Input: part model. Units: mm. Frame: model coordinates. Face numbers are marked on the shaded views. A direction names the side the tool comes from. Give positions to 0.01 mm unless a question says otherwise; leave off trailing zeros. Write each loop counter-clockwise with the first axis right and the second up, starting at its lowest first coordinate (ties: lowest second). Pieces come first, ordered by that corner, then holes.
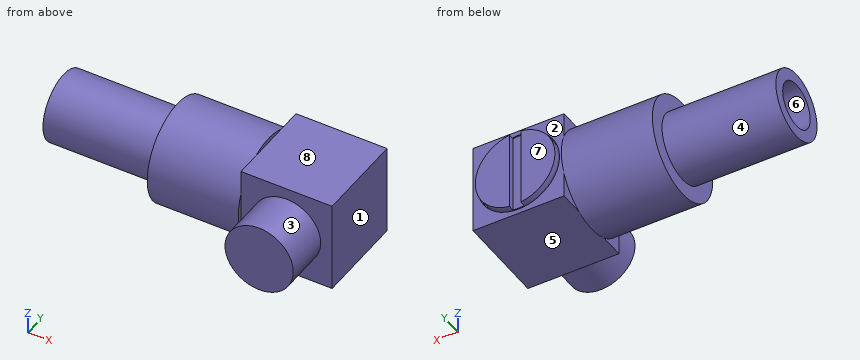
Autodesk Inventor part; units mm, degrees
ref_plane "YZ Plane" through (0, 0, 0) normal (1, 0, 0) x (0, 1, 0)
ref_plane "XZ Plane" through (0, 0, 0) normal (0, 1, 0) x (-1, 0, 0)
ref_plane "XY Plane" through (0, 0, 0) normal (0, 0, 1) x (1, 0, 0)
sketch "Sketch1" plane through (0, 0, 0) normal (0, 1, 0) x (-1, 0, 0)
  line L0 (0, 0) -> (8, 0)
  line L1 (8, 0) -> (8, -4.4)
  line L2 (8, -4.4) -> (0, -4.4)
  line L3 (0, -4.4) -> (0, 0)
  line L4 (0, 0) -> (-8, 0)
  line L5 (-8, 0) -> (-8, -4)
  line L6 (-8, -4) -> (0, -4)
  line L7 (0, -4) -> (0, 0)
  line L8 (-8, 0) -> (0, 0)
  line L9 (0, 0) -> (0, 4)
  line L10 (0, 4) -> (-8, 4)
  line L11 (-8, 4) -> (-8, 0)
  circle A0 centre (-4, 0) radius 3
  line L12 (8, -2) -> (18, -2)
  line L13 (18, -2) -> (18, -3)
  line L14 (18, -3) -> (8, -3)
  line L15 (8, -3) -> (8, -2)
  circle A1 centre (-4, 0) radius 3.5
  line L16 (-3.5, 3.6063) -> (-4.5, 3.6063)
  line L17 (-4.5, 3.6063) -> (-4.5, -3.6063)
  line L18 (-4.5, -3.6063) -> (-3.5, -3.6063)
  line L19 (-3.5, -3.6063) -> (-3.5, 3.6063)
  line L20 (-3.5, 3.6063) -> (-4.5, -3.6063) construction
  line L21 (-4.5, 3.6063) -> (-3.5, -3.6063) construction
  point P0 (-4.5, 3.4641)
  point P1 (-4.5, -3.4641)
  point P2 (-3.5, -3.4641)
  point P3 (-3.5, 3.4641)
  dimension "d0" = 8
  dimension "d1" = 4.4
  dimension "d2" = 8
  dimension "d3" = 4
  dimension "d4" = 4
  dimension "d5" = 6
  dimension "d6" = 10
  dimension "d7" = 1
  dimension "d8" = 2
  dimension "d9" = 7
  dimension "d10" = 1
revolve "Revolution1" add sketch "Sketch1" angle 360 about axis through (0, 0, 0) along (-1, 0, 0) contours L0 L1 L2 L3
revolve "Revolution2" add sketch "Sketch1" angle 360 about axis through (0, 0, 0) along (-1, 0, 0) contours L12 L13 L14 L1
extrude "Extrusion1" add sketch "Sketch1" along normal mid plane 8 contours L3 L6 L5 L4 A1 L17 L18 L19 | L4 A1 L19 L16 L17 L11 L10 L9 | A1 L19 A0 L4 | L4 A0 L19 A1 | A0 L19 L4 | L4 L19 A0 | L19 A0 L17 A1 | A1 L17 L16 L19 | L19 L18 L17 A1 | A1 L17 A0 L19 | L19 A0 L17 L4 | L4 L17 A0 L19 | L17 A0 L4 A1 | A1 L4 A0 L17 | L17 A0 L4 | L4 A0 L17
extrude "Extrusion2" add sketch "Sketch1" against normal blind 8 contours A0 L19 L4 | L4 L19 A0 | L19 A0 L17 L4 | L4 L17 A0 L19 | L17 A0 L4 | L4 A0 L17
extrude "Extrusion3" add sketch "Sketch1" along normal blind 4.5 contours A1 L19 A0 L4 | L4 A0 L19 A1 | A0 L19 L4 | L4 L19 A0 | L17 A0 L4 A1 | A1 L4 A0 L17 | L17 A0 L4 | L4 A0 L17
sketch "Sketch2" plane through (0, 4, 0) normal (0, 1, 0) x (1, 0, 0)
  arc A0 (3.5, 3.4641) -> (3.5, -3.4641) centre (4, 0) ccw
  line L0 (3.5, -3.4641) -> (3.5, 3.4641)
  arc A1 (4.5, -3.4641) -> (4.5, 3.4641) centre (4, 0) ccw
  line L1 (4.5, 3.4641) -> (4.5, -3.4641)
  line L2 (4.5, -3.4641) -> (4.5, 3.4641)
  arc A2 (4.5, -3.4641) -> (4.5, 3.4641) centre (4, 0) ccw
  line L3 (3.5, 3.4641) -> (3.5, -3.4641)
  arc A3 (3.5, 3.4641) -> (3.5, -3.4641) centre (4, 0) ccw
  line L4 (0, -4) -> (8, -4)
  line L5 (8, -4) -> (8, 4)
  line L6 (8, 4) -> (0, 4)
  line L7 (0, 4) -> (0, 1.833)
  line L8 (0, -1.833) -> (0, 1.833)
  line L9 (0, -1.833) -> (0, -4)
  circle A4 centre (4, 0) radius 3.6
  circle A5 centre (4, 0) radius 3.5
  point P0 (0, 0)
  point P1 (3.5, -3.4641)
  dimension "d19" = 7.2
extrude "Extrusion4" cut sketch "Sketch2" against normal blind 0.5 contours A4
thread "Thread1"
properties part number "6mm hose fitting"
Item 1: Ray query, line 1 (Z direction, x = -15.5, y = 0); line 2 (X direction, y = 0, z = 4.25). Return the intervals inside material, ascending.
Item 2: Section A-A (x = 4). Return loops of the section in (y, z), and give its area (3 significant figures).
Item 3: Set-up query: the marked faces 1, 2, 3, 4 and 5. Return all of +Z, -Z, +X, -X, +Y, -Y with unobstructed straight access to the full face (end or side cutting, diameter ignored); none if empty.
Item 4: Section D-D (x = -9.25). Return loops of the section in (y, z).
Item 5: Section C-C (y = 0). Return loops of the section in (x, z).
Item 6: Pin query (flat end, axial travel): pin 1 (1 mm diameter, centred on x = -11, y = 2, fed in from -Z); pin 2 (0.7 mm diameter, centred on y = 3, z = 2.5, fed in from -X); pin 3 (2.5 mm diameter, centred on x = 4.5, y = -0.5, fed in from -Z). Return the tip coordinate at first contact, or that it passes through.
Item 7: Mould query, pull axis Z, two halves, no side actions, for the marked faces 6, 7 and 8. Classes: +Z half, -Z half, draft (parallel to the pull), parting line (faces both ways), or undercut.
Solved:
1. line 1: z = -3 to -2, 2 to 3
1. line 2: x = -8 to 0
2. outline: (-8, -3) - (-4, -3) - (-4, -4) - (4, -4) - (4, -3.6) - (3.5, -3.6) - (3.5, -3.5) - (4, -3.5) - (4, 3.5) - (3.5, 3.5) - (3.5, 3.6) - (4, 3.6) - (4, 4) - (-4, 4) - (-4, 3) - (-8, 3) - close
2. area: 87.9 mm2
3. face 1: +Z, -Z, +X, +Y, -Y
3. face 2: +Y
3. face 3: -Y
3. face 4: -X
3. face 5: -Z, +X, +Y, -Y
4. outline: circle Ø6 at (0, 0); hole circle Ø4 at (0, 0)
5. outline: (-18, -3) - (-8, -3) - (-8, -4.4) - (0, -4.4) - (0, -4) - (8, -4) - (8, 4) - (0, 4) - (0, 4.4) - (-8, 4.4) - (-8, 3) - (-18, 3) - (-18, 2) - (-8, 2) - (-8, -2) - (-18, -2) - close
6. pin 1: stops at z = -2.6
6. pin 2: stops at x = -8
6. pin 3: stops at z = -4
7. face 6: undercut
7. face 7: draft
7. face 8: +Z half
